Geometry: final body of the model. Coordinates: model frame, mm. A direction names the side the tool comes from. Give positions to 0.01 mm unless a question says otherwise; leave off trailing zeros. Write each loop counter-clockwise with the first axis right and the second up, starting at its lowest first coordinate (ties: lowest second). Pieces come first, ordered by that corner, then holes. Notation, with made-up numbers: (81.5, 39.25) -> (136.5, 39.25) arc R24 cw to (136.5, 72.25) -> close; hole circle Ø1 at (-16, -9). An arc over 180 degrees is marked (long way). Use CSV: the item, a comma, the result in double quotes. Start each with the question number.
1) Contact query for flat-ended pins moving along their axis: P1, Ø1.3, axis at x = 145.5, z = 0.5, coming from the -Y side; P2, Ø0.5, axis at y = 101, z = 1, coming from the -X side; P3, Ø12, axis at y = -17, z = 15.5, coming from the +X side; P4, Ø1.7, axis at y = 15.5, z = 1, coming from the -X side. Output: stop coordinate, or through.
2) Section A-A (x = 88.9). Count the separate pieces of the cut face and the enclosed holes in it, plus the area to 3 significant figures.
3) Set-up query: faces 1 (the face through (25.4, -32, 13)), 2 (the face through (75.489, -30.557, 2.263)), 3 (the face through (75, -31.356, 17)), 4 (the face through (127, -32, 13)). Return all of +Z, -Z, +X, -X, +Y, -Y with unobstructed straight access to the full face (end or side cutting, diameter ignored); none if empty.
4) Material intervals for line 1 (X direction, y = -32.05, z = 19.05) (3 decimals); line 2 (Y direction, x = 78.5, z = 11.25); line 3 (Z direction, x = 24.5, y = 25.5), sorted ascending. Write a range as [from, to].
5) Section B-B (z = 5.5). Output: boundary loops of the cut face in (x, y), plus the area to 3 significant figures.
6) Draft query along X for faces 5 (the face through (0.78, 33.73, 19.46)), 6 (the face through (1.562, 44, 17)), 7 (the face through (111.2, -32.14, 18.36)). Return one class per face: pulls with the +X half, pulls with the -X half, needs draft (parallel to the pull), parting line crosses it, or undercut.
```python
from build123d import *

# Parameters (mm, degrees)
BOSS_EXTRUDE1_DEPTH          = 1.5875
SKETCH7_W                    = 1.5875
SKETCH7_H                    = 101.6
BOSS_EXTRUDE2_DEPTH          = 0.0254
EDGE_FLANGE1_STRIP_W         = 19.05
EDGE_FLANGE1_STRIP_H         = 1.5875
EDGE_FLANGE1_STRIP_CUT_DEPTH = 101.6
EDGE_FLANGE1_DEPTH           = 101.6
SKETCH11_W                   = 101.6
SKETCH11_H                   = 1.5875
BOSS_EXTRUDE3_DEPTH          = 0.0254
EDGE_FLANGE2_STRIP_W         = 19.05
EDGE_FLANGE2_STRIP_H         = 1.5875
EDGE_FLANGE2_STRIP_CUT_DEPTH = 101.6
EDGE_FLANGE2_DEPTH           = 101.6
SKETCH15_R                   = 3.175
CUT_EXTRUDE1_DEPTH           = 2.54
SKETCH16_R                   = 3.175
CUT_EXTRUDE2_DEPTH           = 2.54
CUT_EXTRUDE6_DEPTH           = 2.54


# Sheet-metal steps are written as plain solids
with BuildPart() as part:
    # Sketch1 → Boss-Extrude1 (new body)
    with BuildSketch(Plane.XY):
        Polygon((0, 119.481843199), (0, -32.918156801), (152.4, -32.918156801), align=None)
    extrude(amount=BOSS_EXTRUDE1_DEPTH)

    # Sketch7 → Boss-Extrude2 (add)
    with BuildSketch(Plane.ZY):
        with Locations((0.79375, 43.281843199)):
            Rectangle(SKETCH7_W, SKETCH7_H)
    extrude(amount=BOSS_EXTRUDE2_DEPTH)

    # Edge-Flange1 strip (across the edge) → Edge-Flange1 strip cut (cut)
    with BuildSketch(Plane(origin=(-0.0254, 94.081843199, 1.5875), x_dir=(1, 0, 0), z_dir=(0, -1, 0))):
        with Locations((-1.5875, -0.79375)):
            Rectangle(EDGE_FLANGE1_STRIP_W, EDGE_FLANGE1_STRIP_H)
    extrude(amount=EDGE_FLANGE1_STRIP_CUT_DEPTH, mode=Mode.SUBTRACT)

    # Edge-Flange1 section (across the edge) → Edge-Flange1 (add)
    with BuildSketch(Plane(origin=(-0.0254, 94.081843199, 1.5875), x_dir=(1, 0, 0), z_dir=(0, -1, 0))):
        with BuildLine():
            Line((0, 6.35), (0, 23.8125))
            Line((0, 23.8125), (1.5875, 23.8125))
            Line((1.5875, 23.8125), (1.5875, 6.35))
            ThreePointArc((1.5875, 6.35), (3.447371939, 1.859871939), (7.9375, 0))
            Line((7.9375, 0), (7.9375, -1.5875))
            ThreePointArc((7.9375, -1.5875), (2.324839924, 0.737339924), (0, 6.35))
        make_face()
    extrude(amount=EDGE_FLANGE1_DEPTH)

    # Sketch11 → Boss-Extrude3 (add)
    with BuildSketch(Plane(origin=(0, -32.918156801, 0), x_dir=(-1, 0, 0), z_dir=(0, -1, 0))):
        with Locations((-76.2, -0.79375)):
            Rectangle(SKETCH11_W, SKETCH11_H)
    extrude(amount=BOSS_EXTRUDE3_DEPTH)

    # Edge-Flange2 strip (across the edge) → Edge-Flange2 strip cut (cut)
    with BuildSketch(Plane(origin=(25.4, -32.943556801, 1.5875), x_dir=(0, 1, 0), z_dir=(1, 0, 0))):
        with Locations((-1.5875, -0.79375)):
            Rectangle(EDGE_FLANGE2_STRIP_W, EDGE_FLANGE2_STRIP_H)
    extrude(amount=EDGE_FLANGE2_STRIP_CUT_DEPTH, mode=Mode.SUBTRACT)

    # Edge-Flange2 section (across the edge) → Edge-Flange2 (add)
    with BuildSketch(Plane(origin=(25.4, -32.943556801, 1.5875), x_dir=(0, 1, 0), z_dir=(1, 0, 0))):
        with BuildLine():
            Line((0, 6.35), (0, 23.8125))
            Line((0, 23.8125), (1.5875, 23.8125))
            Line((1.5875, 23.8125), (1.5875, 6.35))
            ThreePointArc((1.5875, 6.35), (3.447371939, 1.859871939), (7.9375, 0))
            Line((7.9375, 0), (7.9375, -1.5875))
            ThreePointArc((7.9375, -1.5875), (2.324839924, 0.737339924), (0, 6.35))
        make_face()
    extrude(amount=EDGE_FLANGE2_DEPTH)

    # Sketch15 → Cut-Extrude1 (cut)
    with BuildSketch(Plane(origin=(0, -31.356056801, 0), x_dir=(1, 0, 0), z_dir=(0, 1, 0))):
        with Locations(Location((38.1, -19.05, 0), (0, 0, 270))):
            Circle(SKETCH15_R)
        with Locations(Location((63.5, -19.05, 0), (0, 0, 270))):
            Circle(SKETCH15_R)
        with Locations(Location((88.9, -19.05, 0), (0, 0, 270))):
            Circle(SKETCH15_R)
        with Locations(Location((114.3, -19.05, 0), (0, 0, 270))):
            Circle(SKETCH15_R)
    extrude(amount=-CUT_EXTRUDE1_DEPTH, mode=Mode.SUBTRACT)

    # Sketch16 → Cut-Extrude2 (cut)
    with BuildSketch(Plane(origin=(1.5621, 0, 0), x_dir=(0, 0, -1), z_dir=(1, 0, 0))):
        with Locations((-19.05, 81.381843199)):
            Circle(SKETCH16_R)
        with Locations((-19.05, 55.981843199)):
            Circle(SKETCH16_R)
        with Locations((-19.05, 30.581843199)):
            Circle(SKETCH16_R)
        with Locations((-19.05, 5.181843199)):
            Circle(SKETCH16_R)
    extrude(amount=-CUT_EXTRUDE2_DEPTH, mode=Mode.SUBTRACT)

    # Sketch23 → Cut-Extrude6 (cut)
    with BuildSketch(Plane(origin=(0, 0, 0), x_dir=(-1, 0, 0), z_dir=(0, 0, -1))):
        with BuildLine():
            Line((-54.573395113, 10.50380224), (-49.145810825, 10.50380224))
            ThreePointArc((-49.145810825, 10.50380224), (-46.796706145, 13.083281254), (-48.781433081, 15.952577991))
            add(Edge.make_bspline(
                [(-48.781433081, 15.952577991), (-49.604210691, 16.082970195), (-51.083841149, 16.078342253), (-54.195922097, 16.035293361)],
                knots=[0.430340986, 0.430340986, 0.430340986, 0.430340986, 1, 1, 1, 1], degree=3))
            Line((-54.195922097, 16.035293361), (-61.650359925, 15.903259941))
            Line((-61.650359925, 15.903259941), (-61.746981527, 7.343931221))
            Line((-61.746981527, 7.343931221), (-61.843602617, -1.215397719))
            Line((-61.843602617, -1.215397719), (-65.621203901, -1.215397719))
            Line((-65.621203901, -1.215397719), (-69.398804677, -1.215397719))
            Line((-69.398804677, -1.215397719), (-69.398822965, 10.317171545))
            Line((-69.398822965, 10.317171545), (-69.398822965, 21.849740809))
            Line((-69.398822965, 21.849740809), (-58.122813005, 21.849740809))
            add(Edge.make_bspline(
                [(-58.122813005, 21.849740809), (-47.145028509, 21.849740809), (-46.804351517, 21.828297113), (-45.241678493, 21.038856985)],
                knots=[0, 0, 0, 0, 1, 1, 1, 1], degree=3))
            add(Edge.make_bspline(
                [(-45.241678493, 21.038856985), (-40.484510461, 18.635606521), (-39.407981245, 9.867736325), (-43.424538109, 6.239017141)],
                knots=[0, 0, 0, 0, 1, 1, 1, 1], degree=3))
            add(Edge.make_bspline(
                [(-43.424538109, 6.239017141), (-45.171541981, 4.660705845), (-46.271260381, 4.477914745), (-53.152055357, 4.622150677)],
                knots=[0, 0, 0, 0, 1, 1, 1, 1], degree=3))
            Line((-53.152055357, 4.622150677), (-58.348663709, 4.731083149))
            Line((-58.348663709, 4.731083149), (-60.339924976, 10.364052271))
            add(Edge.make_bspline(
                [(-60.339924976, 10.364052271), (-60.339785544, 10.446289733), (-57.744845223, 10.50917935), (-54.573395113, 10.50380224)],
                knots=[0, 0, 0, 0, 1, 1, 1, 1], degree=3))
        make_face()
        with BuildLine():
            Line((-93.522388131, 1.627502866), (-91.989800897, 4.503859321))
            Line((-91.989800897, 4.503859321), (-86.086398429, 4.617469457))
            add(Edge.make_bspline(
                [(-86.086398429, 4.617469457), (-81.318957113, 4.709221877), (-80.117365409, 4.835103769), (-79.841927301, 5.271672365)],
                knots=[0, 0, 0, 0, 1, 1, 1, 1], degree=3))
            add(Edge.make_bspline(
                [(-79.841927301, 5.271672365), (-79.654305121, 5.569050485), (-79.498376553, 9.419876413), (-79.495340745, 13.831000941)],
                knots=[0, 0, 0, 0, 1, 1, 1, 1], degree=3))
            Line((-79.495340745, 13.831000941), (-79.489821833, 21.849740809))
            Line((-79.489821833, 21.849740809), (-75.705697829, 21.849740809))
            Line((-75.705697829, 21.849740809), (-71.921573317, 21.849740809))
            Line((-71.921573317, 21.849740809), (-71.921573317, 12.352626453))
            add(Edge.make_bspline(
                [(-71.921573317, 12.352626453), (-71.921573317, 3.097047809), (-71.942194053, 2.825210913), (-72.732457141, 1.664079377)],
                knots=[0, 0, 0, 0, 1, 1, 1, 1], degree=3))
            add(Edge.make_bspline(
                [(-72.732457141, 1.664079377), (-73.178443041, 1.008787825), (-74.000851861, 0.133375809), (-74.560031337, -0.281281223)],
                knots=[0, 0, 0, 0, 1, 1, 1, 1], degree=3))
            add(Edge.make_bspline(
                [(-74.560031337, -0.281281223), (-75.523356309, -0.995630315), (-76.087920585, -1.040808787), (-85.315848789, -1.142028803)],
                knots=[0, 0, 0, 0, 1, 1, 1, 1], degree=3))
            Line((-85.315848789, -1.142028803), (-95.054974853, -1.248853075))
            Line((-95.054974853, -1.248853075), (-93.522388131, 1.627502866))
        make_face()
        with BuildLine():
            Line((-39.125829917, 11.921041845), (-39.125829917, 21.849740809))
            Line((-39.125829917, 21.849740809), (-35.708737437, 21.849740809))
            Line((-35.708737437, 21.849740809), (-32.291649021, 21.849740809))
            Line((-32.291649021, 21.849740809), (-32.194909565, 13.470608469))
            Line((-32.194909565, 13.470608469), (-32.098170109, 5.091476129))
            Line((-32.098170109, 5.091476129), (-25.701039901, 4.993059765))
            Line((-25.701039901, 4.993059765), (-19.303905629, 4.894643909))
            Line((-19.303905629, 4.894643909), (-17.862494237, 2.027820585))
            add(Edge.make_bspline(
                [(-17.862494237, 2.027820585), (-17.069717565, 0.451065801), (-16.421082845, -0.923695483), (-16.421082845, -1.027204039)],
                knots=[0, 0, 0, 0, 1, 1, 1, 1], degree=3))
            add(Edge.make_bspline(
                [(-16.421082845, -1.027204039), (-16.421082845, -1.130712595), (-20.759309373, -1.211707099), (-26.061589853, -1.207191487)],
                knots=[0, 0, 0, 0, 1, 1, 1, 1], degree=3))
            add(Edge.make_bspline(
                [(-26.061589853, -1.207191487), (-34.226807965, -1.200233919), (-35.884200637, -1.109240451), (-36.892080765, -0.612529227)],
                knots=[0, 0, 0, 0, 1, 1, 1, 1], degree=3))
            add(Edge.make_bspline(
                [(-36.892080765, -0.612529227), (-39.040522493, 0.446283489), (-39.125829917, 0.924935313), (-39.125829917, 11.921041845)],
                knots=[0, 0, 0, 0, 1, 1, 1, 1], degree=3))
        make_face()
    extrude(amount=-CUT_EXTRUDE6_DEPTH, mode=Mode.SUBTRACT)


solid = part.part
```
Answers follow:
1,P1,"stops at y = -32.92"
1,P2,"stops at x = 0"
1,P3,"passes through"
1,P4,"stops at x = 2.82"
2,separate pieces,"3"
2,enclosed holes,"0"
2,area,"115 mm^2"
3,face 1,"+Z, -X, +Y, -Y"
3,face 2,"-Z, -Y"
3,face 3,"+Z, +X, -X, +Y"
3,face 4,"+Z, +X, +Y, -Y"
4,line 1,"x = [25.4, 34.925], [41.275, 60.325], [66.675, 85.725], [92.075, 111.125], [117.475, 127]"
4,line 2,"y = [-32.94, -31.36]"
4,line 3,"z = [0, 1.59]"
5,outline,"(0.36, -7.52) -> (2.05, -7.52) -> (2.05, 94.08) -> (0.36, 94.08) -> close; (25.4, -32.56) -> (127, -32.56) -> (127, -30.87) -> (25.4, -30.87) -> close"
5,area,"343 mm^2"
6,face 5,"needs draft"
6,face 6,"pulls with the +X half"
6,face 7,"undercut"
